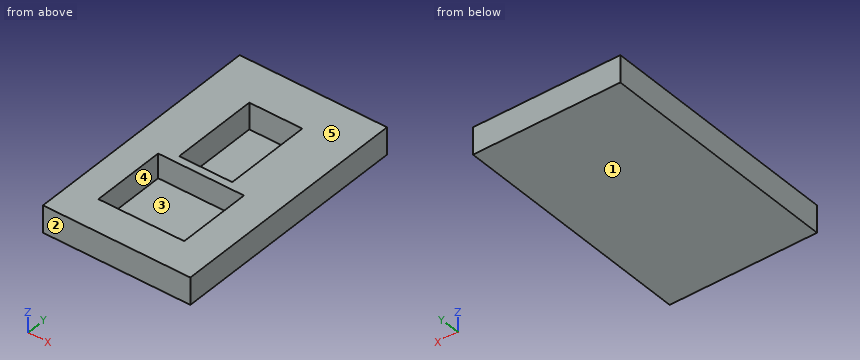
```python
from build123d import *

# Parameters (mm, degrees)
F0_W     = 56.681249
F0_H     = 10.396719
F1_DEPTH = 94.488
F2_W     = 31.195983
F2_H     = 31.680895
F3_DEPTH = 2.54
F4_W     = 20.394963
F4_H     = 33.683496
F5_DEPTH = 10.16
F6_W     = 33.012585
F6_H     = 28.702568
F7_DEPTH = 9.398


with BuildPart() as f1:
    # F0 (on Front) → F1 (new body)
    with BuildSketch(Plane.XZ):
        with Locations((-8.483941, 22.552885)):
            Rectangle(F0_W, F0_H)
    extrude(amount=F1_DEPTH)

    # F2 (on face) → F3 (join)
    with BuildSketch(Plane.XY.offset(27.751245)):
        with Locations((-9.093156, -17.717516)):
            Rectangle(F2_W, F2_H)
    extrude(amount=-F3_DEPTH)

    # F4 (on face) → F5 (cut)
    with BuildSketch(Plane.XY.offset(27.751245)):
        with Locations((-9.785975, -33.244646)):
            Rectangle(F4_W, F4_H)
    extrude(amount=-F5_DEPTH, mode=Mode.SUBTRACT)

    # F6 (on face) → F7 (cut)
    with BuildSketch(Plane.XY.offset(27.751245)):
        with Locations((-9.240382, -67.351179)):
            Rectangle(F6_W, F6_H)
    extrude(amount=-F7_DEPTH, mode=Mode.SUBTRACT)


solid = f1.part
```
Can you work these out from the model? Positions are in its coordinate system, mm. Face numbers are marked on the shaded views. A direction names the side the tool comes from. Round coordinates to 2 decimals unless told otherwise and drop trailing zeros. Loops run counter-clockwise (first coordinate to the right, second up) from the corner with the lowest first, then second, coordinate; pieces in that order, holes last. Notation, with made-up numbers: (82, 17.5) -> (120, 17.5) arc R26 cw to (120, 54.5) -> close; hole circle Ø9 at (21, 67). An arc over 180 degrees is marked (long way). One line per item, written item: value. Start each with the question number.
1. If we section it at C-C, the plane y = -68.5: Write out the boundary of the cut face in (x, z).
2. If we section it at B-B, the plane z = 26.75: Write out the boundary of the cut face in (x, y), then the cut area to 3 significant figures.
3. If we section it at D-D, the plane x = 3: Write out the boundary of the cut face in (y, z).
4. If we mould it in two halves opening along Y, with no side actions, what happens to the marked faces 1, 2 and 3? For each: pulls with the +Y half, pulls with the -Y half, needs draft (parallel to the pull), parting line crosses it, or undercut.
5. If we section it at A-A, the plane x = -14: Write out the boundary of the cut face in (y, z), then the cut area to 3 significant figures.
6. For the marked faces 4 and 5, which set-ups out of +Z, -Z, +X, -X, +Y, -Y let a thin tool reach every point of the face, with its end or its side?
7. If I drill on probe 1 along Y at (x, z) = (-7.5, 20); probe 2 along X at (y, z) = (-22, 21.5); probe 3 along Y at (x, z) = (-22, 26), over which ranges is the centre line in solid material (lowest first)?
Calculated:
1. outline: (-36.82, 17.35) -> (19.86, 17.35) -> (19.86, 27.75) -> (7.27, 27.75) -> (7.27, 18.35) -> (-25.75, 18.35) -> (-25.75, 27.75) -> (-36.82, 27.75) -> close
2. outline: (-36.82, -94.49) -> (19.86, -94.49) -> (19.86, 0) -> (-36.82, 0) -> close; hole (-25.75, -81.7) -> (7.27, -81.7) -> (7.27, -53) -> (-25.75, -53) -> close; hole (-19.98, -50.09) -> (0.41, -50.09) -> (0.41, -16.4) -> (-19.98, -16.4) -> close
2. area: 3,720 mm²
3. outline: (-94.49, 17.35) -> (0, 17.35) -> (0, 27.75) -> (-53, 27.75) -> (-53, 18.35) -> (-81.7, 18.35) -> (-81.7, 27.75) -> (-94.49, 27.75) -> close
4. face 1: needs draft
4. face 2: pulls with the -Y half
4. face 3: undercut
5. outline: (-94.49, 17.35) -> (0, 17.35) -> (0, 27.75) -> (-16.4, 27.75) -> (-16.4, 17.59) -> (-50.09, 17.59) -> (-50.09, 27.75) -> (-53, 27.75) -> (-53, 18.35) -> (-81.7, 18.35) -> (-81.7, 27.75) -> (-94.49, 27.75) -> close
5. area: 370 mm²
6. face 4: +Z
6. face 5: +Z, +X, -X, +Y, -Y
7. probe 1: y = -94.49 to -81.7, -53 to -50.09, -16.4 to 0
7. probe 2: x = -36.82 to -19.98, 0.41 to 19.86
7. probe 3: y = -94.49 to -81.7, -53 to 0
